Build history of the part. All positions in model axes, mm. A direction names the side the tool comes from. Coordinates: 2 decimals unless noted, no trailing zeros. Order: outer loops, then holes, each group sorted by start corner. A loop starts at its lowest first (then second) coordinate and runs counter-clockwise, first axis right, second up. Notation, with made-up numbers: M 68,3 L 103,3 A31 ccw 103,33 Z; hole C 53,11.5 d2. An arc over 180 degrees is marked long. Use a Markdown table: item, result. Add a question column.
Autodesk Fusion 360 part; units mm, degrees
sketch "Sketch1" plane through (0, 0, 0) normal (0, 0, 1) x (1, 0, 0)
  line L0 (-127.0827, 37.5) -> (-102.0827, 37.5)
  line L1 (-102.0827, 37.5) -> (-102.0827, -37.5)
  line L2 (-102.0827, -37.5) -> (-127.0827, -37.5)
  line L3 (0, 0) -> (-132.5, 0) construction
  line L4 (-97.0827, 10) -> (-92.2827, 10)
  line L5 (-92.2827, 10) -> (-92.2827, -10)
  line L6 (-92.2827, -10) -> (-97.0827, -10)
  line L7 (-97.0827, -10) -> (-97.0827, 10)
  arc A0 (-127.0827, 37.5) -> (-132.5, 0) centre (0, 0) ccw construction
  arc A1 (-132.5, 0) -> (-127.0827, -37.5) centre (0, 0) ccw construction
  line L8 (0, 0) -> (66.25, -114.7484) construction
  line L9 (0, 0) -> (66.25, -114.7484) construction
  line L10 (31.0654, -128.8068) -> (18.5654, -107.1562)
  line L11 (18.5654, -107.1562) -> (83.5173, -69.6562)
  line L12 (83.5173, -69.6562) -> (96.0173, -91.3068)
  arc A2 (-127.0827, -37.5) -> (31.0654, -128.8068) centre (0, 0) ccw
  arc A3 (31.0654, -128.8068) -> (66.25, -114.7484) centre (0, 0) ccw construction
  line L13 (37.4811, -84.9191) -> (54.8016, -74.9191)
  line L14 (54.8016, -74.9191) -> (57.2016, -79.076)
  line L15 (57.2016, -79.076) -> (39.8811, -89.076)
  line L16 (39.8811, -89.076) -> (37.4811, -84.9191)
  line L17 (0, 0) -> (132.5, 0) construction
  line L18 (0, 0) -> (66.25, 114.7484) construction
  line L19 (96.0173, 91.3068) -> (83.5173, 69.6562)
  line L20 (83.5173, 69.6562) -> (18.5654, 107.1562)
  line L21 (18.5654, 107.1562) -> (31.0654, 128.8068)
  line L22 (57.2016, 79.076) -> (39.8811, 89.076)
  line L23 (39.8811, 89.076) -> (37.4811, 84.9191)
  line L24 (37.4811, 84.9191) -> (54.8016, 74.9191)
  line L25 (54.8016, 74.9191) -> (57.2016, 79.076)
  circle A4 centre (-115.8879, 45.5) radius 1.5
  circle A5 centre (0, 0) radius 124.5 construction
  circle A6 centre (-115.8879, -45.5) radius 1.5
  circle A7 centre (18.5398, -123.1118) radius 1.5
  circle A8 centre (97.3481, -77.6118) radius 1.5
  circle A9 centre (18.5398, 123.1118) radius 1.5
  line L26 (-102.0827, -18.5) -> (-19.0827, -18.5) construction
  line L27 (-19.0827, -18.5) -> (-19.0827, 18.5) construction
  line L28 (-19.0827, 18.5) -> (-102.0827, 18.5) construction
  line L29 (35.0199, 97.6562) -> (-6.4801, 25.7761) construction
  line L30 (-6.4801, 25.7761) -> (25.5628, 7.2761) construction
  line L31 (25.5628, 7.2761) -> (67.0628, 79.1562) construction
  line L32 (35.0199, -97.6562) -> (-6.4801, -25.7761) construction
  line L33 (-6.4801, -25.7761) -> (25.5628, -7.2761) construction
  line L34 (25.5628, -7.2761) -> (67.0628, -79.1562) construction
  line L35 (-92.0827, 72.5) -> (-21.0827, 72.5) construction
  line L36 (-21.0827, 72.5) -> (-21.0827, 28.5) construction
  line L37 (-21.0827, 28.5) -> (-92.0827, 28.5) construction
  line L38 (-92.0827, 28.5) -> (-92.0827, 72.5) construction
  circle A10 centre (-24.0827, 69.5) radius 1.5
  circle A11 centre (-89.0827, 69.5) radius 1.5
  circle A12 centre (-89.0827, 31.5) radius 1.5
  circle A13 centre (-24.0827, 31.5) radius 1.5
  arc A14 (66.25, -114.7484) -> (96.0173, -91.3068) centre (0, 0) ccw construction
  arc A15 (96.0173, 91.3068) -> (66.25, 114.7484) centre (0, 0) ccw construction
  arc A16 (31.0654, 128.8068) -> (-127.0827, 37.5) centre (0, 0) ccw
  arc A17 (66.25, 114.7484) -> (31.0654, 128.8068) centre (0, 0) ccw construction
  line L39 (125.8662, 41.4) -> (43.6662, 41.4) construction
  line L40 (43.6662, 41.4) -> (43.6662, -41.4) construction
  line L41 (43.6662, -41.4) -> (125.8662, -41.4) construction
  line L42 (43.6662, 13.8) -> (33.1662, 13.8)
  line L43 (33.1662, 13.8) -> (33.1662, 18.6)
  line L44 (33.1662, 18.6) -> (43.6662, 18.6)
  line L45 (68.6662, 36.6) -> (78.2887, 36.6)
  circle A18 centre (97.3481, 77.6118) radius 1.5
  line L46 (104.2763, 73.6118) -> (85.2169, 40.6)
  circle A19 centre (78.2887, 44.6) radius 1.5
  line L47 (43.6662, 13.8) -> (43.6662, -13.8)
  line L48 (43.6662, -13.8) -> (33.1662, -13.8)
  line L49 (33.1662, -13.8) -> (33.1662, -18.6)
  line L50 (33.1662, -18.6) -> (43.6662, -18.6)
  line L51 (68.6662, -36.6) -> (78.2887, -36.6)
  line L52 (104.2763, -73.6118) -> (85.2169, -40.6)
  circle A20 centre (78.2887, -44.6) radius 1.5
  arc A21 (132.5, 0) -> (125.8662, 41.4) centre (0, 0) ccw construction
  arc A22 (103.6034, 82.599) -> (96.0173, 91.3068) centre (0, 0) ccw
  arc A23 (106.9418, 78.2286) -> (103.6034, 82.599) centre (0, 0) ccw construction
  line L53 (106.9418, 78.2286) -> (104.2763, 73.6118) construction
  arc A24 (125.8662, 41.4) -> (106.9418, 78.2286) centre (0, 0) ccw construction
  line L54 (78.2887, 36.6) -> (82.9075, 36.6) construction
  arc A25 (85.2169, 40.6) -> (78.2887, 36.6) centre (78.2887, 44.6) ccw construction
  arc A26 (78.2887, 36.6) -> (85.2169, 40.6) centre (78.2887, 44.6) ccw
  line L55 (85.2169, 40.6) -> (82.9075, 36.6) construction
  line L56 (78.2887, -36.6) -> (82.9075, -36.6) construction
  line L57 (85.2169, -40.6) -> (82.9075, -36.6) construction
  arc A27 (78.2887, -36.6) -> (85.2169, -40.6) centre (78.2887, -44.6) ccw construction
  arc A28 (85.2169, -40.6) -> (78.2887, -36.6) centre (78.2887, -44.6) ccw
  arc A29 (96.0173, -91.3068) -> (103.6034, -82.599) centre (0, 0) ccw
  arc A30 (125.8662, -41.4) -> (132.5, 0) centre (0, 0) ccw construction
  arc A31 (106.9418, -78.2286) -> (125.8662, -41.4) centre (0, 0) ccw construction
  line L58 (106.9418, -78.2286) -> (104.2763, -73.6118) construction
  arc A32 (103.6034, -82.599) -> (106.9418, -78.2286) centre (0, 0) ccw construction
  arc A33 (104.2763, -73.6118) -> (103.6034, -82.599) centre (97.3481, -77.6118) ccw construction
  arc A34 (103.6034, -82.599) -> (104.2763, -73.6118) centre (97.3481, -77.6118) ccw
  arc A35 (103.6034, 82.599) -> (104.2763, 73.6118) centre (97.3481, 77.6118) ccw construction
  arc A36 (104.2763, 73.6118) -> (103.6034, 82.599) centre (97.3481, 77.6118) ccw
  line L59 (33.1662, 13.8) -> (33.1662, -13.8) construction
  line L60 (48.6662, 41.4) -> (48.6662, 36.6)
  line L61 (68.6662, 41.4) -> (68.6662, 36.6)
  line L62 (48.6662, 36.6) -> (43.6662, 36.6)
  line L63 (43.6662, 18.6) -> (43.6662, 36.6)
  line L64 (50.6662, 41.4) -> (50.6662, 45.4)
  line L65 (50.6662, 45.4) -> (56.6662, 45.4)
  line L66 (56.6662, 45.4) -> (56.6662, 41.4)
  circle A37 centre (60.6662, 46.4) radius 1.5
  line L67 (48.6662, 41.4) -> (50.6662, 41.4)
  line L68 (56.6662, 41.4) -> (68.6662, 41.4)
  line L69 (43.6662, -36.6) -> (48.6662, -36.6)
  line L70 (48.6662, -36.6) -> (48.6662, -41.4)
  line L71 (48.6662, -41.4) -> (50.6662, -41.4)
  line L72 (50.6662, -41.4) -> (50.6662, -45.4)
  line L73 (50.6662, -45.4) -> (56.6662, -45.4)
  line L74 (56.6662, -45.4) -> (56.6662, -41.4)
  line L75 (56.6662, -41.4) -> (68.6662, -41.4)
  line L76 (68.6662, -41.4) -> (68.6662, -36.6)
  line L77 (43.6662, -18.6) -> (43.6662, -36.6)
  circle A38 centre (60.6662, -46.4) radius 1.5
  circle A39 centre (12.9173, 0) radius 1.5
  point P0 (-102.0827, 0)
  point P1 (-97.0827, 0)
  point P2 (51.0413, -88.4062)
  point P3 (48.5413, -84.076)
  point P4 (51.0413, 88.4062)
  point P5 (48.5413, 84.076)
  point P6 (-19.0827, 0)
  point P7 (9.5413, 16.5261)
  point P8 (9.5413, -16.5261)
  point P9 (43.6662, 0)
  point P10 (53.6662, 45.4)
  point P11 (53.6662, -45.4)
  point P12 (12.9173, 0)
  dimension "d1" = 265
  dimension "d2" = 75
  dimension "d3" = 25
  dimension "d4" = 4.8
  dimension "d5" = 20
  dimension "d6" = 5
  dimension "d17" = 120
  dimension "d19" = 132.5
  dimension "d20" = 75
  dimension "d21" = 25
  dimension "d22" = 20
  dimension "d23" = 4.8
  dimension "d24" = 5
  dimension "d25" = 132.5
  dimension "d28" = 60
  dimension "d29" = 75
  dimension "d30" = 25
  dimension "d31" = 4.8
  dimension "d32" = 20
  dimension "d33" = 5
  dimension "d34" = 3
  dimension "d35" = 8
  dimension "d36" = 249
  dimension "d37" = 3
  dimension "d38" = 8
  dimension "d39" = 3
  dimension "d40" = 8
  dimension "d41" = 3
  dimension "d42" = 8
  dimension "d49" = 3
  dimension "d50" = 8
  dimension "d53" = 37
  dimension "d55" = 37
  dimension "d57" = 78
  dimension "d58" = 78
  dimension "d59" = 37
  dimension "d60" = 78
  dimension "d61" = 71
  dimension "d62" = 44
  dimension "d63" = 10
  dimension "d64" = 10
  dimension "d75" = 3
  dimension "d76" = 3
  dimension "d77" = 3
  dimension "d78" = 3
  dimension "d85" = 3
  dimension "d86" = 3
  dimension "d87" = 3
  dimension "d88" = 3
  dimension "d89" = 3
  dimension "d90" = 3
  dimension "d91" = 3
  dimension "d92" = 3
  dimension "d156" = 82.8
  dimension "d157" = 82.2
  dimension "d161" = 4.8
  dimension "d162" = 13.8
  dimension "d167" = 3
  dimension "d168" = 8
  dimension "d169" = 8
  dimension "d170" = 3
  dimension "d171" = 8
  dimension "d172" = 8
  dimension "d173" = 10.5
  dimension "d174" = 4.8
  dimension "d175" = 27.6
  dimension "d180" = 8
  dimension "d181" = 3
  dimension "d182" = 8
  dimension "d183" = 8
  dimension "d184" = 4.8
  dimension "d185" = 4.8
  dimension "d186" = 20
  dimension "d187" = 5
  dimension "d188" = 4
  dimension "d189" = 6
  dimension "d190" = 10
  dimension "d191" = 3
  dimension "d193" = 17
  dimension "d194" = 5
  dimension "d195" = 4.8
  dimension "d196" = 5
  dimension "d197" = 6
  dimension "d198" = 4
  dimension "d199" = 10
  dimension "d200" = 20
  dimension "d201" = 3
  dimension "d202" = 5
  dimension "d203" = 17
  dimension "d204" = 4.8
  dimension "d205" = 115
  dimension "d206" = 3
extrude "Extrude1" add sketch "Sketch1" against normal blind 4.8
(1) Drill centre lines: line 1 along X through (y, z) = (9.5, -1.05); line 2 along Y through (x, z) = (51, -0.8); line 3 along X through (y, z) = (17, -3.4). Where is each one in solid material? Low to high. Write a range as from..to.
(2) Slice it at B-B on y = 96.5. Give the cut face in (x, z), and give its area (3 significant figures).
(3) Drop flat-ended pins along their axis: P1, Ø1.4, axis at y = -17.5, z = -3, coming from the +X side; P2, Ø2.5, axis at x = 37.5, z = -2.5, coming from the -Y side; P3, Ø1.5, axis at x = -30.5, z = -2.5, coming from the +Y side; P4, Ø5, axis at x = -115.89, y = 45.5, coming from the -Z side. Give the stop position or say it passes through.
(4) Slice it at A-A on z = -1.6. State how many separate pieces and enclosed holes the cut face has, and give its area (3 significant figures).
(5) Which spindle directions (+Z, -Z, +X, -X, +Y, -Y) get a long thin tool onto all of the face, cutting with end or side? Do faces 5 (the flat face through (50.587, -88.669, -2.366)), 6 (the flat face through (94.88, -57.34, -2.37)), 7 (the flat face through (-12, 2, 0)). Say none if no direction does.
(6) Mould opens along Y. For faces 1 (the flat face through (89.855, 80.633, -2.366)), 2 (the flat face through (51.5, 88.14, -2.37)), 3 (the flat face through (-12, 2, -4.8)), 4 (the flat face through (89.68, -80.33, -2.37)) say: released by +Y, released by -Y, zero draft, split by the parting line, or undercut.
(7) Slice it at C-C on y = -55. Give the cut face in (x, z).
Solutions:
| question | item | result |
|---|---|---|
| 1 | line 1 | -102.08..-97.08, -92.28..43.67 |
| 1 | line 2 | -88.43..-82.66, -77.11..-45.4, 45.4..77.11, 82.66..88.43 |
| 1 | line 3 | -102.08..33.17 |
| 2 | outline | M -90.8,-4.8 L 37.02,-4.8 L 37.02,0 L -90.8,0 Z |
| 2 | area | 614 mm² |
| 3 | P1 | x = 33.17 |
| 3 | P2 | y = -96.95 |
| 3 | P3 | y = 129.12 |
| 3 | P4 | z = -4.8 |
| 4 | separate pieces | 1 |
| 4 | enclosed holes | 18 |
| 4 | area | 39,600 mm² |
| 5 | face 5 | +Z, -Z |
| 5 | face 6 | +Z, -Z, +X |
| 5 | face 7 | +Z, +X, -X, +Y, -Y |
| 6 | face 1 | released by +Y |
| 6 | face 2 | undercut |
| 6 | face 3 | zero draft |
| 6 | face 4 | released by -Y |
| 7 | outline | M -120.55,-4.8 L 93.53,-4.8 L 93.53,0 L -120.55,0 Z |
